Answer from the drawing. Dimensions are ordinates in mm from the lowest x, y and z of the part. Round coordinates to 2 decimals unless told otherwise and drop trailing zeros. Loops run counter-clockwise (first coordinate to the right, second up) from the corner with the lowest first, then second, coordinate; pieces in that order, holes last.
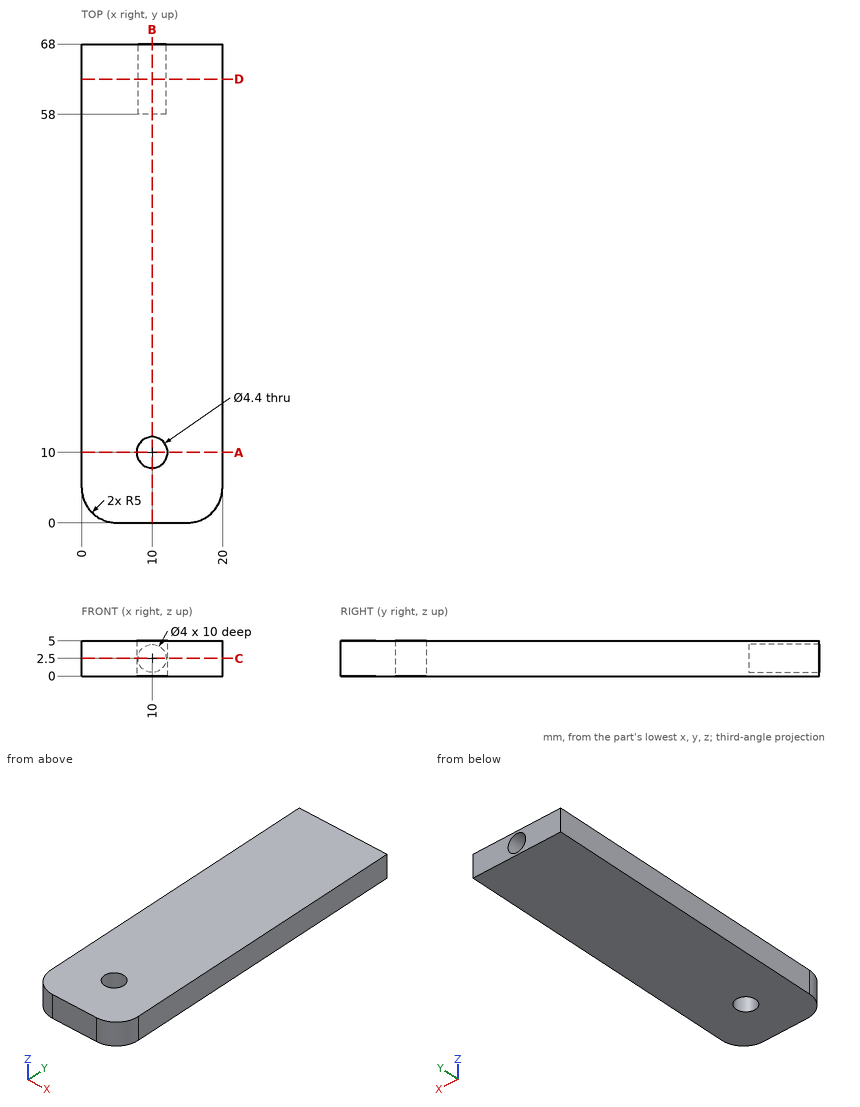
1. Given pin 1 (4 mm diameter, centred on x = 10, y = 10, fed in from -Z); pin 2 (1.2 mm diameter, centred on x = 10, z = 2, fed in from +Y); pin 3 (1.5 mm diameter, centred on x = 3.5, z = 2, fed in from -Y), each flat-ended and moving along its own axis, determine where each tip first touches the part or whether it passes through.
Answer key:
pin 1: passes through
pin 2: stops at y = 58
pin 3: stops at y = 0.06
2. Find section A-A (y = 10). Write down the section's boundary in (x, z), then the cut area to 3 significant figures.
Answer key:
outline: (0, 0) - (7.8, 0) - (7.8, 5) - (0, 5) - close; (12.2, 0) - (20, 0) - (20, 5) - (12.2, 5) - close
area: 78.0 mm2
3. Consider probe 1 along Y at (x, z) = (10, 1.05); probe 2 along Z at (x, y) = (11.5, 64.5); probe 3 along X at (y, z) = (64, 1.35). Determine where each line is inside the solid, lowest interval first.
Answer key:
probe 1: y = 0 to 7.8, 12.2 to 58
probe 2: z = 0 to 1.18, 3.82 to 5
probe 3: x = 0 to 8.36, 11.64 to 20
4. Find section D-D (y = 63). Write down the section's boundary in (x, z).
Answer key:
outline: (0, 0) - (20, 0) - (20, 5) - (0, 5) - close; hole circle Ø4 at (10, 2.5)
5. Find section B-B (x = 10). Write down the section's boundary in (y, z), then the cut area to 3 significant figures.
Answer key:
outline: (0, 0) - (7.8, 0) - (7.8, 5) - (0, 5) - close; (12.2, 0) - (68, 0) - (68, 0.5) - (58, 0.5) - (58, 4.5) - (68, 4.5) - (68, 5) - (12.2, 5) - close
area: 278 mm2
6. Find section C-C (z = 2.5). Write down the section's boundary in (x, y).
Answer key:
outline: (0, 5) arc R5 ccw to (5, 0) - (15, 0) arc R5 ccw to (20, 5) - (20, 68) - (12, 68) - (12, 58) - (8, 58) - (8, 68) - (0, 68) - close; hole circle Ø4.4 at (10, 10)
